Build history of the part. All positions in model axes, mm. Coordinates: 2 decimals unless noted, no trailing zeros.
(1) Wall check: L1, parallel to X at y = -2, z = -131.5; L2, parallel to Y at x = 6.5, z = -43; L3, parallel to Y at x = 5.25, z = -268. Give the ranges that are in metal, low to high.
(2) Slice it at A-A (z = -93.5). Give the number of separate pieces and of enclosed holes in the cut face, and give its area (3 significant figures).
(3) Flat gauge pins, fed straight in: P1, Ø1.6, axis at y = -0.5, z = -251.5, coming from the +X side; P2, Ø2.5, axis at y = -5.5, z = -253.5, coming from the -X side; P3, Ø1.1, axis at y = 5.5, z = -136, coming from the -X side. Where does each tip first touch, or does it go through?
(4) Two-plate mould, pull along X, no slides. Class faces 1 (the face through (0, 3, -355.6)), 2 (the face through (-5.425, -5.689, -175.311)), 3 (the face through (12.7, -8, -175)): pulls with the +X half, pulls with the -X half, needs draft (parallel to the pull), parting line crosses it, or undercut.
from build123d import *

# Parameters (mm, degrees)
EXTRUDE1_DEPTH = 355.6


with BuildPart() as part:
    # Sketch2 → Extrude1 (new body)
    with BuildSketch(Plane.XY):
        with BuildLine():
            Line((-4.3561, 12.7), (-10.5918, 12.7))
            ThreePointArc((-10.5918, 12.7), (-12.082522516, 12.082522516), (-12.7, 10.5918))
            Line((-12.7, 10.5918), (-12.7, 6.35))
            ThreePointArc((-12.7, 6.35), (-7.120384182, -7.120384182), (6.35, -12.7))
            Line((6.35, -12.7), (10.5918, -12.7))
            ThreePointArc((10.5918, -12.7), (12.082522516, -12.082522516), (12.7, -10.5918))
            Line((12.7, -10.5918), (12.7, -4.3561))
            ThreePointArc((12.7, -4.3561), (11.5951, -3.2512), (10.4902, -4.3561))
            Line((10.4902, -4.3561), (10.4902, -6.474899798))
            ThreePointArc((10.4902, -6.474899798), (9.863006367, -7.413561403), (8.75577951, -7.193320288))
            Line((8.75577951, -7.193320288), (5.447103113, -3.88464389))
            ThreePointArc((5.447103113, -3.88464389), (4.758849627, -2.854599758), (4.517167143, -1.63957986))
            Line((4.517167143, -1.63957986), (4.517167143, 1.63957986))
            ThreePointArc((4.517167143, 1.63957986), (4.758849627, 2.854599758), (5.447103113, 3.88464389))
            Line((5.447103113, 3.88464389), (8.75577951, 7.193320288))
            ThreePointArc((8.75577951, 7.193320288), (9.863006367, 7.413561403), (10.4902, 6.474899798))
            Line((10.4902, 6.474899798), (10.4902, 4.3561))
            ThreePointArc((10.4902, 4.3561), (11.5951, 3.2512), (12.7, 4.3561))
            Line((12.7, 4.3561), (12.7, 10.5918))
            ThreePointArc((12.7, 10.5918), (12.082522516, 12.082522516), (10.5918, 12.7))
            Line((10.5918, 12.7), (4.3561, 12.7))
            ThreePointArc((4.3561, 12.7), (3.2512, 11.5951), (4.3561, 10.4902))
            Line((4.3561, 10.4902), (6.474899798, 10.4902))
            ThreePointArc((6.474899798, 10.4902), (7.413561403, 9.863006367), (7.193320288, 8.75577951))
            Line((7.193320288, 8.75577951), (3.88464389, 5.447103113))
            ThreePointArc((3.88464389, 5.447103113), (2.854599758, 4.758849627), (1.63957986, 4.517167143))
            Line((1.63957986, 4.517167143), (-1.63957986, 4.517167143))
            ThreePointArc((-1.63957986, 4.517167143), (-2.854599758, 4.758849627), (-3.88464389, 5.447103113))
            Line((-3.88464389, 5.447103113), (-7.193320288, 8.75577951))
            ThreePointArc((-7.193320288, 8.75577951), (-7.413561403, 9.863006367), (-6.474899798, 10.4902))
            Line((-6.474899798, 10.4902), (-4.3561, 10.4902))
            ThreePointArc((-4.3561, 10.4902), (-3.2512, 11.5951), (-4.3561, 12.7))
        make_face()
        with BuildLine():
            Line((-1.340533428, -2.231856263), (-1.969151357, -2.860474191))
            ThreePointArc((-1.969151357, -2.860474191), (-2.918583239, -2.918583239), (-2.860474191, -1.969151357))
            Line((-2.860474191, -1.969151357), (-2.231856263, -1.340533428))
            ThreePointArc((-2.231856263, -1.340533428), (-2.6035, 0), (-2.231856263, 1.340533428))
            Line((-2.231856263, 1.340533428), (-2.860474191, 1.969151357))
            ThreePointArc((-2.860474191, 1.969151357), (-2.918583239, 2.918583239), (-1.969151357, 2.860474191))
            Line((-1.969151357, 2.860474191), (-1.340533428, 2.231856263))
            ThreePointArc((-1.340533428, 2.231856263), (0, 2.6035), (1.340533428, 2.231856263))
            Line((1.340533428, 2.231856263), (1.969151357, 2.860474191))
            ThreePointArc((1.969151357, 2.860474191), (2.918583239, 2.918583239), (2.860474191, 1.969151357))
            Line((2.860474191, 1.969151357), (2.231856263, 1.340533428))
            ThreePointArc((2.231856263, 1.340533428), (2.6035, 0), (2.231856263, -1.340533428))
            Line((2.231856263, -1.340533428), (2.860474191, -1.969151357))
            ThreePointArc((2.860474191, -1.969151357), (2.918583239, -2.918583239), (1.969151357, -2.860474191))
            Line((1.969151357, -2.860474191), (1.340533428, -2.231856263))
            ThreePointArc((1.340533428, -2.231856263), (0, -2.6035), (-1.340533428, -2.231856263))
        make_face(mode=Mode.SUBTRACT)
        with BuildLine():
            Line((3.884538548, -5.447103113), (7.192726697, -8.755291262))
            ThreePointArc((7.192726697, -8.755291262), (7.414487708, -9.858828287), (6.482287344, -10.489680404))
            ThreePointArc((6.482287344, -10.489680404), (-5.557819617, -5.557819617), (-10.489680404, 6.482287344))
            ThreePointArc((-10.489680404, 6.482287344), (-9.858828287, 7.414487708), (-8.755291262, 7.192726697))
            Line((-8.755291262, 7.192726697), (-5.447103113, 3.884538548))
            ThreePointArc((-5.447103113, 3.884538548), (-4.758849627, 2.854494415), (-4.517167143, 1.639474517))
            Line((-4.517167143, 1.639474517), (-4.517167143, -2.307367143))
            ThreePointArc((-4.517167143, -2.307367143), (-3.869931708, -3.869931708), (-2.307367143, -4.517167143))
            Line((-2.307367143, -4.517167143), (1.639474517, -4.517167143))
            ThreePointArc((1.639474517, -4.517167143), (2.854494415, -4.758849627), (3.884538548, -5.447103113))
        make_face(mode=Mode.SUBTRACT)
    extrude(amount=-EXTRUDE1_DEPTH)


solid = part.part
Response values:
1. L1: x = -10.77 to -8.27, -4.52 to -2.9, 2.9 to 4.54
1. L2: y = -12.7 to -10.49, -8.06 to -4.94, 4.94 to 8.06, 10.49 to 12.7
1. L3: y = -12.67 to -10.45, -6.81 to -3.67, 3.67 to 6.81, 10.49 to 12.7
2. separate pieces: 1
2. enclosed holes: 2
2. area: 271 mm2
3. P1: stops at x = 4.52
3. P2: stops at x = -9.48
3. P3: stops at x = -12.7
4. face 1: needs draft
4. face 2: undercut
4. face 3: pulls with the +X half
